Geometry: final body of the model. Coordinates: model frame, mm. Coordinates: 2 decimals unless noted, no trailing zeros. Write each loop counter-clockwise with the first axis right and the second up, starting at its lowest first coordinate (ties: lowest second). Pieces come first, ordered by that corner, then holes. Notation, with made-up numbers: (49, -4) -> (104, -4) arc R16 ccw to (104, 8) -> close; hole circle Ø10 at (-16, 56). An arc over 180 degrees is marked (long way). Answer as a JSON object with one key per item and string values. Group by question number.
```python
from build123d import *

# Parameters (mm, degrees)
SKETCH1_W                   = 508
SKETCH1_H                   = 965.2
BOSS_EXTRUDE1_DEPTH         = 3.81
F_1_16_1_2_DIAMETER_HOLE1_D = 30.48
CHAMFER1_SIZE               = 101.6
CUT_EXTRUDE2_DEPTH          = 4.81


with BuildPart() as part:
    # Sketch1 → Boss-Extrude1 (new body)
    with BuildSketch(Plane.XY):
        Rectangle(SKETCH1_W, SKETCH1_H)
    extrude(amount=BOSS_EXTRUDE1_DEPTH)

    # 1/16 (1.2) Diameter Hole1 (through all)
    with Locations(Plane.XY.offset(3.81)):
        with Locations((-190.5, 254), (190.5, 254), (190.5, -254), (-190.5, -254)):
            Hole(F_1_16_1_2_DIAMETER_HOLE1_D / 2)

    # Chamfer1
    chamfer1_edges = [part.edges().sort_by_distance(p)[0] for p in [
        (-254, 482.6, 1.905),
        (-254, -482.6, 1.905),
        (254, -482.6, 1.905),
        (254, 482.6, 1.905),
    ]]
    chamfer(chamfer1_edges, length=CHAMFER1_SIZE)

    # Sketch6 → Cut-Extrude2 (cut, through all)
    with BuildSketch(Plane.XY.offset(3.81)):
        Polygon((-63.5, 431.8), (63.5, 431.8), (139.7, 355.6), (139.7, 50.8), (-139.7, 50.8), (-139.7, 355.6), align=None)
        Polygon((139.7, -355.6), (139.7, -50.8), (-139.7, -50.8), (-139.7, -355.6), (-63.5, -431.8), (63.5, -431.8), align=None)
    extrude(amount=-CUT_EXTRUDE2_DEPTH, mode=Mode.SUBTRACT)


solid = part.part
```
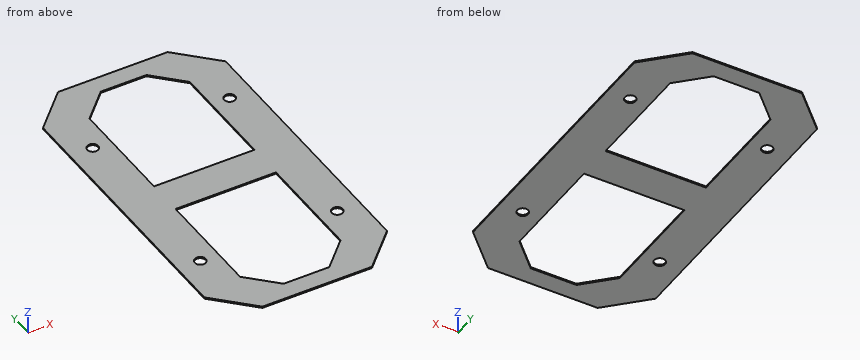
Item 1: Contact query for flat-ended pins moving along their axis: pin 1 (24.5 mm diameter, centred on x = 190.5, y = -254, fed in from +Z); pin 2 (10 mm diameter, centred on x = -89.5, y = 44.5, fed in from -Z). Output: stop coordinate, or through.
Item 2: Section D-D on y = -370. Output: boundary loops of the cut face in (x, z), then the cut area to 3 significant figures.
Item 3: Section C-C on z = 0.6. Output: boundary loops of the cut face in (x, y).
Item 4: Ray query, L1, parallel to Y at x = 4.5, z = 3.55; L2, parallel to X at y = 293.5, z = 1.35; L3, parallel to Y at x = 190.5, z = 1.7. Return the intervals inside material, ascending. Write a range as [from, to].
Item 5: Section A-A on x = -30. Output: boundary loops of the cut face in (y, z), then the cut area to 3 significant figures.
Item 6: Section B-B on y = 254. Output: boundary loops of the cut face in (x, z).
Answer sheet:
{
 "1": {"pin 1": "passes through", "pin 2": "stops at z = 0"},
 "2": {"outline": "(-254, 0) -> (-125.3, 0) -> (-125.3, 3.81) -> (-254, 3.81) -> close; (125.3, 0) -> (254, 0) -> (254, 3.81) -> (125.3, 3.81) -> close", "area": "981 mm^2"},
 "3": {"outline": "(-254, -381) -> (-152.4, -482.6) -> (152.4, -482.6) -> (254, -381) -> (254, 381) -> (152.4, 482.6) -> (-152.4, 482.6) -> (-254, 381) -> close; hole circle Ø30.48 at (-190.5, -254); hole circle Ø30.48 at (-190.5, 254); hole (-139.7, -355.6) -> (-63.5, -431.8) -> (63.5, -431.8) -> (139.7, -355.6) -> (139.7, -50.8) -> (-139.7, -50.8) -> close; hole (-139.7, 50.8) -> (139.7, 50.8) -> (139.7, 355.6) -> (63.5, 431.8) -> (-63.5, 431.8) -> (-139.7, 355.6) -> close; hole circle Ø30.48 at (190.5, -254); hole circle Ø30.48 at (190.5, 254)"},
 "4": {"L1": "y = [-482.6, -431.8], [-50.8, 50.8], [431.8, 482.6]", "L2": "x = [-254, -139.7], [139.7, 254]", "L3": "y = [-444.5, -269.24], [-238.76, 238.76], [269.24, 444.5]"},
 "5": {"outline": "(-482.6, 0) -> (-431.8, 0) -> (-431.8, 3.81) -> (-482.6, 3.81) -> close; (-50.8, 0) -> (50.8, 0) -> (50.8, 3.81) -> (-50.8, 3.81) -> close; (431.8, 0) -> (482.6, 0) -> (482.6, 3.81) -> (431.8, 3.81) -> close", "area": "774 mm^2"},
 "6": {"outline": "(-254, 0) -> (-205.74, 0) -> (-205.74, 3.81) -> (-254, 3.81) -> close; (-175.26, 0) -> (-139.7, 0) -> (-139.7, 3.81) -> (-175.26, 3.81) -> close; (139.7, 0) -> (175.26, 0) -> (175.26, 3.81) -> (139.7, 3.81) -> close; (205.74, 0) -> (254, 0) -> (254, 3.81) -> (205.74, 3.81) -> close"}
}
